```python
from build123d import *

# Parameters (mm, degrees)
CROQUIS4_W              = 104
CROQUIS4_H              = 104
CROQUIS4_R              = 1.85
SALIENTE_EXTRUIR2_DEPTH = 6
CROQUIS5_R              = 2.85
CROQUIS5_R_2            = 1.85
SALIENTE_EXTRUIR3_DEPTH = 5
REDONDEO1_R             = 2
REDONDEO2_R             = 1
SALIENTE_EXTRUIR4_DEPTH = 3


with BuildPart() as part:
    # Croquis4 → Saliente-Extruir2 (new body)
    with BuildSketch(Plane.XY):
        Rectangle(CROQUIS4_W, CROQUIS4_H)
        with Locations((-46.5, 46.3)):
            Circle(CROQUIS4_R, mode=Mode.SUBTRACT)
        with Locations((46.5, 46.9)):
            Circle(CROQUIS4_R, mode=Mode.SUBTRACT)
        with Locations((-46.4, -46.6)):
            Circle(CROQUIS4_R, mode=Mode.SUBTRACT)
        with Locations((46.2, -46.7)):
            Circle(CROQUIS4_R, mode=Mode.SUBTRACT)
    extrude(amount=SALIENTE_EXTRUIR2_DEPTH)

    # Croquis5 → Saliente-Extruir3 (add)
    with BuildSketch(Plane.XY.offset(6)):
        with Locations((-46.5, 46.3)):
            Circle(CROQUIS5_R)
        with Locations((-46.5, 46.3)):
            Circle(CROQUIS5_R_2, mode=Mode.SUBTRACT)
        with Locations((46.5, 46.9)):
            Circle(CROQUIS5_R)
        with Locations((46.5, 46.9)):
            Circle(CROQUIS5_R_2, mode=Mode.SUBTRACT)
        with Locations((46.2, -46.7)):
            Circle(CROQUIS5_R)
        with Locations((46.2, -46.7)):
            Circle(CROQUIS5_R_2, mode=Mode.SUBTRACT)
        with Locations((-46.4, -46.6)):
            Circle(CROQUIS5_R)
        with Locations((-46.4, -46.6)):
            Circle(CROQUIS5_R_2, mode=Mode.SUBTRACT)
    extrude(amount=SALIENTE_EXTRUIR3_DEPTH)

    # Redondeo1
    redondeo1_edges = [part.edges().sort_by_distance(p)[0] for p in [
        (43.65, 46.9, 6),
        (-49.35, 46.3, 6),
        (-49.25, -46.6, 6),
        (43.35, -46.7, 6),
    ]]
    fillet(redondeo1_edges, radius=REDONDEO1_R)

    # Redondeo2
    redondeo2_edges = [part.edges().sort_by_distance(p)[0] for p in [
        (-52, 52, 3),
        (52, 52, 3),
        (52, -52, 3),
        (-52, -52, 3),
    ]]
    fillet(redondeo2_edges, radius=REDONDEO2_R)

    # Croquis6 → Saliente-Extruir4 (add)
    with BuildSketch(Plane(origin=(0, 0, 0), x_dir=(-1, 0, 0), z_dir=(0, 0, -1))):
        with BuildLine():
            Line((51, 55), (-51, 55))
            ThreePointArc((-51, 55), (-53.828427125, 53.828427125), (-55, 51))
            Line((-55, 51), (-55, -51))
            ThreePointArc((-55, -51), (-53.828427125, -53.828427125), (-51, -55))
            Line((-51, -55), (51, -55))
            ThreePointArc((51, -55), (53.828427125, -53.828427125), (55, -51))
            Line((55, -51), (55, 51))
            ThreePointArc((55, 51), (53.828427125, 53.828427125), (51, 55))
        make_face()
        with BuildLine():
            Line((-52, 51), (-52, -51))
            ThreePointArc((-52, -51), (-51.707106781, -51.707106781), (-51, -52))
            Line((-51, -52), (51, -52))
            ThreePointArc((51, -52), (51.707106781, -51.707106781), (52, -51))
            Line((52, -51), (52, 51))
            ThreePointArc((52, 51), (51.707106781, 51.707106781), (51, 52))
            Line((51, 52), (-51, 52))
            ThreePointArc((-51, 52), (-51.707106781, 51.707106781), (-52, 51))
        make_face(mode=Mode.SUBTRACT)
    extrude(amount=-SALIENTE_EXTRUIR4_DEPTH)


solid = part.part
```
CAD build for the part. Positions are in the model's coordinates, mm. A direction names the side the tool comes from. Round coordinates to 2 decimals unless told otherwise and drop trailing zeros. Order: outer loops, then holes, each group sorted by start corner. A loop starts at its lowest first (then second) coordinate and runs counter-clockwise, first axis right, second up. Notation, with made-up numbers: (11, 77) - (62, 77) arc R30 ccw to (62, 103) - close; hole circle Ø10 at (42.5, 4). An arc over 180 degrees is marked (long way). Use CSV: the item, a comma, the result in double quotes. Start each with the question number.
1) Pin check, flat tips, straight feed: pin 1 Ø2.5 at (y, z) = (24, 5) entering from +X; pin 2 Ø2 at (x, y) = (-46.4, -46.6) entering from +Z; pin 3 Ø0.9 at (x, z) = (18, 4.5) entering from -Y; pin 4 Ø6 at (x, y) = (-43.5, -11) entering from +Z. Stop position of each tip, or through.
2) Two-plate mould, pull along Y, no slides. Class faces 1 (the flat face through (-1, 52, 4)), 2 (the flat face through (4, -53, 3)), 3 (the cylindrical face through (-47.02, -49.38, 9.48)), 4 (the cylindrical face through (-44.968, 48.703, 9.479)): pulls with the +Y half, pulls with the -Y half, needs draft (parallel to the pull), parting line crosses it, or undercut.
3) Wall check: L1, parallel to Y at x = 46.2, z = 5.25; L2, parallel to Y at x = 46.5, z = 8.25; L3, parallel to Y at x = -46.4, z = 8.5. Give the ranges that are in metal, low to high. Write a range as [from, to].
4) Saw through at C-C (x = -46.5). Count the separate pieces of the cut face and the enclosed holes in it, and give its area (3 significant figures).
5) Tool access for faces 5 (the flat face through (-52, -1, 4)), 6 (the flat face through (-1, -52, 4)), 7 (the cylindrical face through (47.815, 44.372, 9.479)): list every direction of +Z, -Z, +X, -X, +Y, -Y with a clear straight run to the whole face (end or side of a thin tool).
6) Saw through at A-A (y = 33.5). List the corners of the cut face in (x, z).
Values follow:
1,pin 1,"stops at x = 52"
1,pin 2,"passes through"
1,pin 3,"stops at y = -52"
1,pin 4,"stops at z = 6"
2,face 1,"pulls with the +Y half"
2,face 2,"needs draft"
2,face 3,"undercut"
2,face 4,"undercut"
3,L1,"y = [-52, -48.55], [-44.85, 45.07], [48.73, 52]"
3,L2,"y = [-49.53, -48.53], [-44.87, -43.87], [44.05, 45.05], [48.75, 49.75]"
3,L3,"y = [-49.45, -48.45], [-44.75, -43.75], [43.45, 44.45], [48.15, 49.15]"
4,separate pieces,"3"
4,enclosed holes,"0"
4,area,"621 mm2"
5,face 5,"+Z, -X, +Y, -Y"
5,face 6,"+Z, +X, -X, -Y"
5,face 7,"+Z"
6,outline,"(-55, 0) - (55, 0) - (55, 3) - (52, 3) - (52, 6) - (-52, 6) - (-52, 3) - (-55, 3) - close"
